The model under review builds one solid part; all positions refer to its coordinate system, in mm. Round coordinates to 2 decimals unless told otherwise and drop trailing zeros. Loops run counter-clockwise (first coordinate to the right, second up) from the corner with the lowest first, then second, coordinate; pieces in that order, holes last. Notation, with made-up numbers: (9, 33.25) -> (17, 33.25) arc R14 ccw to (17, 56.25) -> close; hole circle Ø7 at (60, 58). An arc over 180 degrees is marked (long way). Write each question's results on one line, items separated by ' | '. Start each with the question number.
Item 1: For L1, parallel to Y at x = 16.37, z = -0.8; L2, parallel to X at y = 0.4, z = -1.35; L3, parallel to Y at x = 15.5, z = -2.45, list the stretches that pass through material, from the lowest coordinate up. Write a range as from..to.
Item 2: Clearance check with a flat-ended pin moving along its axis: pin 1 Ø2.5 at (x, y) = (0, 0) entering from +Z. State where the tip first meets the part, or that it passes through.
Item 3: Mouldability with a two-part tool opening along Y and no side actions: class faces 1 (the cylindrical face through (19.37, 0.07, -0.04)), 2 (the flat face through (8, 0, -3)), 3 (the cylindrical face through (-1.5, 0.07, -0.04)) as pulls with the +Y half, pulls with the -Y half, needs draft (parallel to the pull), parting line crosses it, or undercut.
Item 4: We need section D-D (y = -1.8). Give the boundary of the cut face in (x, z), and give its area (3 significant figures).
Item 5: We need section A-A (y = 0). Give the boundary of the cut face in (x, z), and give its area (3 significant figures).
Item 6: We need section C-C (x = 0.5). Give the boundary of the cut face in (y, z).
Item 7: We need section B-B (z = 1). Give the boundary of the cut face in (x, y), and give its area (3 significant figures).
from build123d import *

# Parameters (mm, degrees)
BOSS_EXTRU_1_DEPTH      = 3
BOSS_EXTRU_1_DEPTH_BACK = 3
ESQUISSE1_R             = 1.5


with BuildPart() as part:
    # Esquisse1 → Boss.-Extru.1 (new, two sides: drawn at the far end of the back side and taken through both)
    with BuildSketch(Plane.XY.offset(-BOSS_EXTRU_1_DEPTH_BACK)):
        with BuildLine():
            Line((0, 3), (16.37, 3))
            ThreePointArc((16.37, 3), (19.37, 0), (16.37, -3))
            Line((16.37, -3), (0, -3))
            ThreePointArc((0, -3), (-3, 0), (0, 3))
        make_face()
        Circle(ESQUISSE1_R, mode=Mode.SUBTRACT)
        with Locations((16.37, 0)):
            Circle(ESQUISSE1_R, mode=Mode.SUBTRACT)
    extrude(amount=BOSS_EXTRU_1_DEPTH + BOSS_EXTRU_1_DEPTH_BACK)


solid = part.part
Here are the results:
1) L1: y = -3..-1.5, 1.5..3 | L2: x = -2.97..-1.45, 1.45..14.92, 17.82..19.34 | L3: y = -3..-1.22, 1.22..3
2) pin 1: passes through
3) face 1: parting line crosses it | face 2: needs draft | face 3: undercut
4) outline: (-2.4, -3) -> (18.77, -3) -> (18.77, 3) -> (-2.4, 3) -> close | area: 127 mm2
5) outline: (-3, -3) -> (-1.5, -3) -> (-1.5, 3) -> (-3, 3) -> close; (1.5, -3) -> (14.87, -3) -> (14.87, 3) -> (1.5, 3) -> close; (17.87, -3) -> (19.37, -3) -> (19.37, 3) -> (17.87, 3) -> close | area: 98.2 mm2
6) outline: (-3, -3) -> (-1.41, -3) -> (-1.41, 3) -> (-3, 3) -> close; (1.41, -3) -> (3, -3) -> (3, 3) -> (1.41, 3) -> close
7) outline: (0, -3) -> (16.37, -3) arc R3 ccw to (16.37, 3) -> (0, 3) arc R3 ccw to start; hole circle Ø3 at (0, 0); hole circle Ø3 at (16.37, 0) | area: 112 mm2
